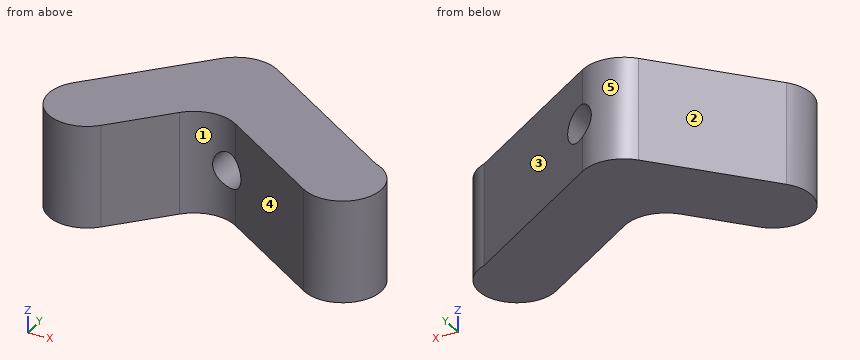
```python
from build123d import *

# Parameters (mm, degrees)
F1_DEPTH = 6.35
F2_R     = 5.08
F3_R     = 2.159
F4_DEPTH = 17.286523


with BuildPart() as f1:
    # F0 (on Top) → F1 (new body, symmetric)
    with BuildSketch(Plane.XY):
        with BuildLine():
            Line((-4.284978, 18.774289), (-18.370262, 3.193811))
            ThreePointArc((-18.370262, 3.193811), (-18.031229, -3.532843), (-11.304576, -3.193811))
            Line((-11.304576, -3.193811), (-2.490694, 6.55569))
            Line((-2.490694, 6.55569), (14.380764, -4.033771))
            ThreePointArc((14.380764, -4.033771), (20.623101, -2.98554), (20.310992, 3.336497))
            Line((20.310992, 3.336497), (18.439706, 4.511019))
            Line((18.439706, 4.511019), (-4.284978, 18.774289))
        make_face()
        with BuildLine():
            ThreePointArc((20.310992, 3.336497), (19.444399, 4.033771), (18.439706, 4.511019))
            Line((18.439706, 4.511019), (20.310992, 3.336497))
        make_face()
    extrude(amount=F1_DEPTH, both=True)

    # F2
    f2_edges = [f1.edges().sort_by_distance(p)[0] for p in [
        (-4.284978, 18.774289, 0),
        (-2.490694, 6.55569, 0),
    ]]
    fillet(f2_edges, radius=F2_R)

    # F3 (on Front) → F4 (cut, through all)
    with BuildSketch(Plane.XZ):
        Circle(F3_R)
    extrude(amount=-F4_DEPTH, mode=Mode.SUBTRACT)


solid = f1.part
```
Design review of the part built by this model. Coordinates are the model's own, in mm. Face numbers are marked on the shaded views. A direction names the side the tool comes from. Give positions to 0.01 mm unless a question says otherwise; leave off trailing zeros. Order: outer loops, then holes, each group sorted by start corner. A loop starts at its lowest first (then second) coordinate and runs counter-clockwise, first axis right, second up. Notation, with made-up numbers: (23, -37.75) - (29, -37.75) arc R7 ccw to (29, -25.75) - close; hole circle Ø4 at (-35.5, 65). An arc over 180 degrees is marked (long way). Use a Markdown table: item, result. Add a question column.
(1) Mouldability with a two-part tool opening along X and no side actions: class the marked faces 1, 2 and 3 as +X half, -X half, draft (parallel to the pull), parting line (faces both ways), or undercut.
(2) Wall thickness on probe 1 along Z at (x, y) = (0, 7.25); probe 2 along X at (y, z) = (14.25, 0); probe 3 along X at (y, z) = (2.75, 1): over which ranges is each line inside the solid? List them lowest first. Write a range as [from, to].
(3) Machinability: for the marked faces 4 and 5, which of the approach directions +Z, -Z, +X, -X, +Y, -Y give a long, thin tool a straight path to every point of the face, cutting with its end or side? Answer none if there is none.
(4) Add section C-C on z = -5. Give the boundary of the cut face in (x, y) (1 decimal), then the cut area to 3 significant figures.
(5) Add section B-B on x = 0. Give the boundary of the cut face in (y, z).
(6) Add section A-A on y = 0. Give the boundary of the cut face in (x, z).
(7) Add section D-D on y = 7.75. Give the boundary of the cut face in (x, z).
(8) Clearance check with flat-ended pins moving along their axes: P1, Ø2.5, axis at x = 0, z = 0, coming from the +Y side; P2, Ø4, axis at y = 7.5, z = 3.5, coming from the -X side; P3, Ø3, axis at y = 5.5, z = -3, coming from the +X side. State where each tip first meets the part, or that it passes through.
Report:
| question | item | result |
|---|---|---|
| 1 | face 1 | undercut |
| 1 | face 2 | -X half |
| 1 | face 3 | +X half |
| 2 | probe 1 | z = [-6.35, -2.16], [2.16, 6.35] |
| 2 | probe 2 | x = [-8.38, -2.16], [2.16, 2.92] |
| 2 | probe 3 | x = [-18.73, -5.93], [3.57, 20.8] |
| 3 | face 4 | +Z, -Z, -Y |
| 3 | face 5 | +Z, -Z, +Y |
| 4 | outline | (-18.4, 3.2) arc R4.8 ccw to (-11.3, -3.2) - (-5.3, 3.4) arc R5.1 cw to (1.1, 4.3) - (14.4, -4) arc R4.8 ccw to (20.3, 3.3) arc R4.8 ccw to (18.4, 4.5) - (-0.7, 16.5) arc R5.1 ccw to (-7.1, 15.6) - close |
| 4 | area | 459 mm² |
| 5 | outline | (4.81, -6.35) - (16.08, -6.35) - (16.08, -2.16) - (4.81, -2.16) - close; (4.81, 2.16) - (16.08, 2.16) - (16.08, 6.35) - (4.81, 6.35) - close |
| 6 | outline | (-19.6, -6.35) - (-8.42, -6.35) - (-8.42, 6.35) - (-19.6, 6.35) - close; (7.95, -6.35) - (21.68, -6.35) - (21.68, 6.35) - (7.95, 6.35) - close |
| 7 | outline | (-14.25, -6.35) - (13.28, -6.35) - (13.28, 6.35) - (-14.25, 6.35) - close; hole circle Ø4.32 at (0, 0) |
| 8 | P1 | passes through |
| 8 | P2 | stops at x = -16.29 |
| 8 | P3 | stops at x = 19.5 |
